Check sheet for the modelled part. Datum: model origin and axes. Units: mm. Face numbers are marked on the shaded views. A direction names the side the tool comes from. Round coordinates to 2 decimals unless told otherwise and drop trailing zeros. Write each loop counter-clockwise with the first axis right and the second up, starting at its lowest first coordinate (ties: lowest second). Pieces come first, ordered by that corner, then holes. Notation, with made-up numbers: M 23,12 L 76,12 A22 cw 76,40 Z; hole C 68,39.25 d10. An arc over 180 degrees is marked long. Put each result on its own line as item: value.
```python
from build123d import *

# Parameters (mm, degrees)
ESQUISSE1_W        = 30
ESQUISSE1_H        = 15
ESQUISSE1_R        = 2.5
BOSS_EXTRU_2_DEPTH = 5
ESQUISSE2_W        = 10
ESQUISSE2_H        = 15
BOSS_EXTRU_3_DEPTH = 10
ESQUISSE3_W        = 10
ESQUISSE3_H        = 7
BOSS_EXTRU_5_DEPTH = 25
BOSS_EXTRU_6_DEPTH = 20
ESQUISSE4_W        = 10
ESQUISSE4_H        = 5
BOSS_EXTRU_7_DEPTH = 18
CONG_1_R           = 10
CONG_2_R           = 3


with BuildPart() as part:
    # Esquisse1 → Boss.-Extru.2 (new body)
    with BuildSketch(Plane.XY):
        Rectangle(ESQUISSE1_W, ESQUISSE1_H)
        with Locations((-10, 0)):
            Circle(ESQUISSE1_R, mode=Mode.SUBTRACT)
        with Locations(Location((10, 0, 0), (0, 0, 180))):
            Circle(ESQUISSE1_R, mode=Mode.SUBTRACT)
    extrude(amount=BOSS_EXTRU_2_DEPTH)

    # Esquisse2 → Boss.-Extru.3 (add)
    with BuildSketch(Plane.XY.offset(5)):
        Rectangle(ESQUISSE2_W, ESQUISSE2_H)
    extrude(amount=BOSS_EXTRU_3_DEPTH)

    # Esquisse3 → Boss.-Extru.5 (add)
    with BuildSketch(Plane(origin=(0, 7.5, 0), x_dir=(1, 0, 0), z_dir=(0, 1, 0))):
        with Locations((0, -11.5)):
            Rectangle(ESQUISSE3_W, ESQUISSE3_H)
    extrude(amount=BOSS_EXTRU_5_DEPTH)

    # Esquisse3_4 → Boss.-Extru.6 (add)
    with BuildSketch(Plane(origin=(0, 7.5, 0), x_dir=(1, 0, 0), z_dir=(0, 1, 0))):
        with BuildLine():
            ThreePointArc((-5, -8), (0, -6.397674733), (5, -8))
            Line((5, -8), (-5, -8))
        make_face()
    extrude(amount=BOSS_EXTRU_6_DEPTH)

    # Esquisse4 → Boss.-Extru.7 (add)
    with BuildSketch(Plane(origin=(0, 0, 8), x_dir=(-1, 0, 0), z_dir=(0, 0, -1))):
        with Locations((0, 30)):
            Rectangle(ESQUISSE4_W, ESQUISSE4_H)
    extrude(amount=BOSS_EXTRU_7_DEPTH)

    # Cong_1
    cong_1_edges = [part.edges().sort_by_distance(p)[0] for p in [
        (0, -7.5, 15),
        (0, 32.5, 15),
    ]]
    fillet(cong_1_edges, radius=CONG_1_R)

    # Cong_2
    cong_2_edges = [part.edges().sort_by_distance(p)[0] for p in [
        (0, 7.5, 6.397674733),
        (0, 27.5, 6.397674733),
    ]]
    fillet(cong_2_edges, radius=CONG_2_R)

    # Sym_trie3: part across plane


with BuildPart() as part_1:
    add(part.part)
    add(part.part.mirror(Plane(origin=(0, 0, -10), x_dir=(1, 0, 0), z_dir=(0, 0, -1))))


solid = part_1.part
```
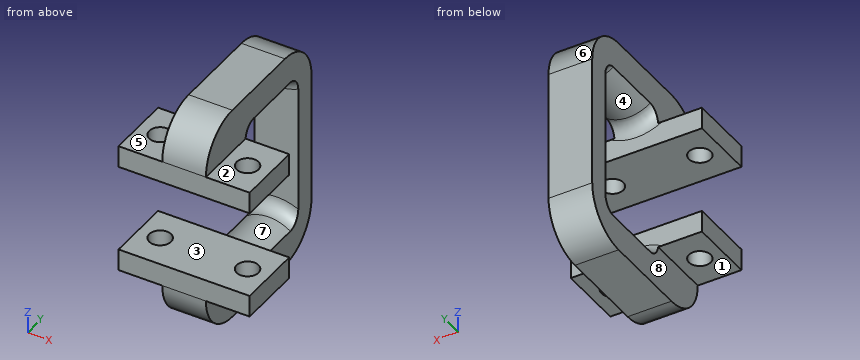
1. Release check for a two-part mould opening along Y. For the marked faces 6, 7 and 8 record: +Y half, -Y half, draft (parallel to the pull), parting line (faces both ways), or undercut.
Computed values:
face 6: +Y half
face 7: undercut
face 8: draft
2. Cross-section at B-B (z = 1). Enter the section's corners in (x, y), then the cut area to 3 significant figures.
Computed values:
outline: M -15,-7.5 L 15,-7.5 L 15,7.5 L -15,7.5 Z; M -5,27.5 L 5,27.5 L 5,32.5 L -5,32.5 Z; hole C -10,0 d5; hole C 10,0 d5
area: 461 mm2
3. Scan lines: probe 1 along Y at (x, z) = (10, 3); probe 2 along Z at (x, y) = (-3, 3); probe 3 along Z at (x, y) = (-12, 3.5). Record each from-to range of solid material in increasing order.
Computed values:
probe 1: y = -7.5 to -2.5, 2.5 to 7.5
probe 2: z = -35 to -20, 0 to 15
probe 3: z = -25 to -20, 0 to 5
4. Access from +Z, -Z, +X, -X, +Y, -Y to the whole of each face (thin tool, end or side, straight path). Record for the marked faces 1, 2, 3, 4 and 5.
Computed values:
face 1: -Z, -X, +Y, -Y
face 2: +Z, +X, +Y, -Y
face 3: +X, -X, -Y
face 4: none
face 5: +Z, -X, +Y, -Y
5. Depth check by flat-ended pin: pin 1 Ø1.5 at (x, y) = (0.5, -1) entering from +Z; pin 2 Ø8 at (x, y) = (10, 0) entering from +Z; pin 3 Ø3 at (x, y) = (-10, -1.5) entering from -Z; pin 4 Ø1.5 at (y, z) = (9, -20) entering from +X. Enter the tip coordinate at first touch or a pass-through.
Computed values:
pin 1: stops at z = 14.61
pin 2: stops at z = 5
pin 3: stops at z = -25
pin 4: passes through
6. Cross-section at C-C (y = 16). Enter the section's corners in (x, z), then the cut area to 3 significant figures.
Computed values:
outline: M -5,-35 L 5,-35 L 5,-28 A8.6 ccw -5,-28 Z; M -5,8 A8.6 ccw 5,8 L 5,15 L -5,15 Z
area: 162 mm2
7. Cross-section at D-D (y = 0). Count the separate pieces of the cut face and the enclosed holes in it, then the cut area to 3 significant figures.
Computed values:
separate pieces: 6
enclosed holes: 0
area: 394 mm2
8. Cross-section at A-A (x = -10). Enter the section's corners in (y, z).
Computed values:
outline: M -7.5,-25 L -2.5,-25 L -2.5,-20 L -7.5,-20 Z; M -7.5,0 L -2.5,0 L -2.5,5 L -7.5,5 Z; M 2.5,-25 L 7.5,-25 L 7.5,-20 L 2.5,-20 Z; M 2.5,0 L 7.5,0 L 7.5,5 L 2.5,5 Z
